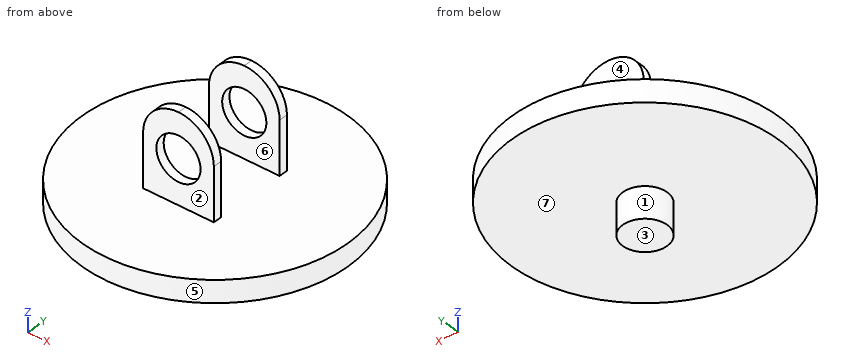
from build123d import *

# Parameters (mm, degrees)
SKETCH1_R           = 25
BOSS_EXTRUDE1_DEPTH = 35
SKETCH2_R           = 150
BOSS_EXTRUDE2_DEPTH = 25
SKETCH3_W           = 80
SKETCH3_H           = 10
BOSS_EXTRUDE3_DEPTH = 100
SKETCH4_R           = 25
CUT_EXTRUDE1_DEPTH  = 297.816441593
FILLET1_R           = 40


with BuildPart() as part:
    # Sketch1 → Boss-Extrude1 (new body)
    with BuildSketch(Plane.XY):
        Circle(SKETCH1_R)
    extrude(amount=BOSS_EXTRUDE1_DEPTH)

    # Sketch2 → Boss-Extrude2 (add)
    with BuildSketch(Plane.XY.offset(35)):
        Circle(SKETCH2_R)
    extrude(amount=BOSS_EXTRUDE2_DEPTH)

    # Sketch3 → Boss-Extrude3 (add)
    with BuildSketch(Plane.XY.offset(60)):
        with Locations((0, -45)):
            Rectangle(SKETCH3_W, SKETCH3_H)
        with Locations((0, 45)):
            Rectangle(SKETCH3_W, SKETCH3_H)
    extrude(amount=BOSS_EXTRUDE3_DEPTH)

    # Sketch4 → Cut-Extrude1 (cut, through all)
    with BuildSketch(Plane.XZ.offset(50)):
        with Locations(Location((0, 110, 0), (0, 0, 90))):
            Circle(SKETCH4_R)
    extrude(amount=-CUT_EXTRUDE1_DEPTH, mode=Mode.SUBTRACT)

    # Fillet1
    fillet1_edges = [part.edges().sort_by_distance(p)[0] for p in [
        (40, -45, 160),
        (40, 45, 160),
        (-40, 45, 160),
        (-40, -45, 160),
    ]]
    fillet(fillet1_edges, radius=FILLET1_R - 0.0001)  # a hair under: the kernel refuses the full size


solid = part.part
Read the model definition and answer for the solid it produces. Units are mm, in the model's axes. Face numbers are marked on the shaded views. A direction names the side the tool comes from. Coordinates: 2 decimals unless noted, no trailing zeros. Loops run counter-clockwise (first coordinate to the right, second up) from the corner with the lowest first, then second, coordinate; pieces in that order, holes last.
Q1. The part is cut by section C-C on x = -18. Write down the section's boundary in (y, z), and give its area (3 significant figures).
Q2. Each of these flat-tipped pins is pushed along its axis until it touches: pin 1 Ø6 at (x, z) = (-18, 143) entering from -Y; pin 2 Ø3 at (y, z) = (-43.5, 98.5) entering from +X; pin 3 Ø8 at (y, z) = (-53, 34.5) entering from +X. Where does it stop, or does it pass through?
Q3. The part is cut by section D-D on z = 149. Write down the section's boundary in (x, y), and give its area (3 significant figures).
Q4. The mould has two halves that part along Y. Classify the marked faces 4, 5, 6 and 7: +Y half, -Y half, draft (parallel to the pull), parting line (faces both ways), or undercut.
Q5. Consider probe 1 along X at (y, z) = (45, 110); probe 2 along Z at (x, y) = (-73, 107.5); probe 3 along X at (y, z) = (-1, 49). Determine where each line is inside the solid, lowest interval first.
Q6. Which of the six approach directions +Z, -Z, +X, -X, +Y, -Y give full straight-line access (tool end or side, diameter ignored) to the marked faces 1, 2 and 3?
Q7. The part is cut by section A-A on z = 110. Write down the section's boundary in (x, y), and give its area (3 significant figures).
Q8. The part is cut by section B-B on y = 0. Write down the section's boundary in (x, z).
Results below:
1. outline: (-148.92, 35) - (-17.35, 35) - (-17.35, 0) - (17.35, 0) - (17.35, 35) - (148.92, 35) - (148.92, 60) - (50, 60) - (50, 92.65) - (40, 92.65) - (40, 60) - (-40, 60) - (-40, 92.65) - (-50, 92.65) - (-50, 60) - (-148.92, 60) - close; (-50, 127.35) - (-40, 127.35) - (-40, 155.72) - (-50, 155.72) - close; (40, 127.35) - (50, 127.35) - (50, 155.72) - (40, 155.72) - close
1. area: 9,880 mm2
2. pin 1: stops at y = -50
2. pin 2: stops at x = 40
2. pin 3: stops at x = 141.76
3. outline: (-27.55, -50) - (27.55, -50) - (27.55, -40) - (-27.55, -40) - close; (-27.55, 40) - (27.55, 40) - (27.55, 50) - (-27.55, 50) - close
3. area: 1,100 mm2
4. face 4: +Y half
4. face 5: parting line
4. face 6: undercut
4. face 7: draft
5. probe 1: x = -40 to -25, 25 to 40
5. probe 2: z = 35 to 60
5. probe 3: x = -150 to 150
6. face 1: -Z
6. face 2: +Z, +X, -X, -Y
6. face 3: -Z, +X, -X, +Y, -Y
7. outline: (-40, -50) - (-25, -50) - (-25, -40) - (-40, -40) - close; (-40, 40) - (-25, 40) - (-25, 50) - (-40, 50) - close; (25, -50) - (40, -50) - (40, -40) - (25, -40) - close; (25, 40) - (40, 40) - (40, 50) - (25, 50) - close
7. area: 600 mm2
8. outline: (-150, 35) - (-25, 35) - (-25, 0) - (25, 0) - (25, 35) - (150, 35) - (150, 60) - (-150, 60) - close
